from build123d import *

# Parameters (mm, degrees)
SKETCH1_R           = 25.4
BOSS_EXTRUDE1_DEPTH = 20.32
SKETCH2_R           = 14.2875
CUT_EXTRUDE1_DEPTH  = 6.35
CUT_EXTRUDE2_START  = -17.78
SKETCH3_R           = 25.4
SKETCH3_R_2         = 16.51
CUT_EXTRUDE2_DEPTH  = 17.78
SKETCH6_R           = 8.763
CUT_EXTRUDE3_DEPTH  = 39.5419369
FILLET1_R           = 1.5875


with BuildPart() as part:
    # Sketch1 → Boss-Extrude1 (new body)
    with BuildSketch(Plane.XY):
        Circle(SKETCH1_R)
    extrude(amount=BOSS_EXTRUDE1_DEPTH)

    # Sketch2 → Cut-Extrude1 (cut)
    with BuildSketch(Plane.XY.offset(20.32)):
        Circle(SKETCH2_R)
    extrude(amount=-CUT_EXTRUDE1_DEPTH, mode=Mode.SUBTRACT)

    # Sketch3 → Cut-Extrude2 (cut)
    with BuildSketch(Plane.XY.offset(20.32).offset(CUT_EXTRUDE2_START)):
        Circle(SKETCH3_R)
        Circle(SKETCH3_R_2, mode=Mode.SUBTRACT)
    extrude(amount=CUT_EXTRUDE2_DEPTH, mode=Mode.SUBTRACT)

    # Sketch5 → Revolve1 (revolve)
    with BuildSketch(Plane(origin=(0, 0, 0), x_dir=(1, 0, 0), z_dir=(0, 1, 0)), mode=Mode.PRIVATE) as revolve1_sk:
        with BuildLine():
            Line((-25.4, -2.54), (-16.51, -2.54))
            Line((-16.51, -2.54), (-16.51, -20.32))
            ThreePointArc((-16.51, -20.32), (-18.869673356, -10.387336678), (-25.4, -2.54))
        make_face()
    revolve(revolve1_sk.sketch.rotate(Axis((0, 0, 0), (0, 0, -1)), 180), axis=Axis((0, 0, 0), (0, 0, -1)))

    # Sketch6 → Cut-Extrude3 (cut, through all)
    with BuildSketch(Plane.XY.offset(13.97)):
        Circle(SKETCH6_R)
    extrude(amount=-CUT_EXTRUDE3_DEPTH, mode=Mode.SUBTRACT)

    # Fillet1
    fillet1_edges = [part.edges().sort_by_distance(p)[0] for p in [
        (-25.4, 0, 2.54),
        (-16.51, 0, 20.32),
        (-25.4, 0, 0),
    ]]
    fillet(fillet1_edges, radius=FILLET1_R)


solid = part.part
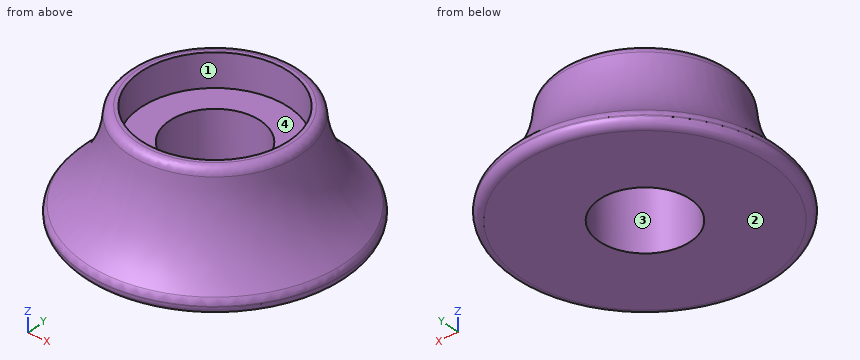
Can you work these out from the model? Positions are in its coordinate system, mm. Face numbers are marked on the shaded views. A direction names the side the tool comes from. Give positions to 0.01 mm unless a question says otherwise; leave off trailing zeros. Loops run counter-clockwise (first coordinate to the right, second up) from the corner with the lowest first, then second, coordinate; pieces in that order, holes last. Notation, with made-up numbers: (-34, 5.25) - (15, 5.25) arc R8 ccw to (15, 18.25) - close; hole circle Ø1 at (-29.75, 35). An arc over 180 degrees is marked (long way). Return JSON: item names as keys, results as strings.
1. I'm going to push flat-ended pins straight in: pin 1 Ø10.5 at (x, y) = (0, 0) entering from +Z; pin 2 Ø5 at (y, z) = (3.5, 12) entering from +X; pin 3 Ø4 at (x, y) = (5.5, -5) entering from +Z; pin 4 Ø5 at (x, y) = (13, 12) entering from +Z. Where does each tip first touch, or does it pass through?
Output values:
{"pin 1": "passes through", "pin 2": "stops at x = 19.08", "pin 3": "stops at z = 13.97", "pin 4": "stops at z = 20.31"}
2. I want a section at B-B on z = 11.25. Please give me the cut outline in (x, y), and give its area (3 significant figures).
Output values:
{"outline": "circle Ø36.92 at (0, 0); hole circle Ø17.53 at (0, 0)", "area": "829 mm²"}
3. We'd pull the mould along Y, two halves only. Please class the marked faces 1 and 2: +Y half, -Y half, draft (parallel to the pull), parting line (faces both ways), or undercut.
Output values:
{"face 1": "undercut", "face 2": "draft"}
4. I want a section at A-A on z = 16. Please give me the cut outline in (x, y) (1 decimal), and give its area (3 significant figures).
Output values:
{"outline": "circle Ø33.9 at (0, 0); hole circle Ø28.6 at (0, 0)", "area": "261 mm²"}
5. If I drill on line 1 (Z direction, x = 1, y = -12.5); line 2 (X direction, y = 9.5, z = 14.5); line 3 (Y direction, x = 0, z = 15.5), over which ranges is the centre line in solid material (lowest first)?
Output values:
{"line 1": "z = 0 to 13.97", "line 2": "x = -14.46 to -10.67, 10.67 to 14.46", "line 3": "y = -17.05 to -14.29, 14.29 to 17.05"}
6. For the marked faces 3 and 4, which set-ups out of +Z, -Z, +X, -X, +Y, -Y let a thin tool reach every point of the face, with its end or its side?
Output values:
{"face 3": "+Z, -Z", "face 4": "+Z"}
